Part model, mm, in its own coordinate system. A direction names the side the tool comes from. Coordinates: 2 decimals unless noted, no trailing zeros. Order: outer loops, then holes, each group sorted by start corner. A loop starts at its lowest first (then second) coordinate and runs counter-clockwise, first axis right, second up.
from build123d import *

# Parameters (mm, degrees)
BOSS_EXTRUDE1_DEPTH               = 2
BOSS_EXTRUDE2_DEPTH               = 4
BOSS_EXTRUDE3_DEPTH               = 1
BOSS_EXTRUDE4_DEPTH               = 3
SKETCH7_W                         = 13
SKETCH7_H                         = 25
CUT_EXTRUDE2_DEPTH                = 0.75
F_3_0_3_DIAMETER_HOLE1_D          = 3
SKETCH12_W                        = 0.5
SKETCH12_H                        = 1.222432211
F_1_0_1_DIAMETER_HOLE1_AT_2_COUNT = 2
F_1_0_1_DIAMETER_HOLE1_AT_2_PITCH = 2
F_1_0_1_DIAMETER_HOLE2_D          = 1
F_1_0_1_DIAMETER_HOLE2_DEPTH      = 3
SKETCH18_W                        = 25
SKETCH18_H                        = 13
CUT_EXTRUDE4_DEPTH                = 10
SKETCH19_W                        = 25
SKETCH19_H                        = 13
CUT_EXTRUDE5_DEPTH                = 62.758096635
SKETCH20_W                        = 0.67
SKETCH20_H                        = 16.929710607
BOSS_EXTRUDE5_DEPTH               = 3
F_1_0_1_DIAMETER_HOLE3_D          = 1
F_1_0_1_DIAMETER_HOLE3_DEPTH      = 3


with BuildPart() as part:
    # Sketch1 → Boss-Extrude1 (new body)
    with BuildSketch(Plane(origin=(0, 0, 0), x_dir=(1, 0, 0), z_dir=(0, 1, 0))):
        Polygon((17.5, 42.5), (-39, 42.5), (-39, 17.5), (-44.5, 17.5), (-44.5, -17.5), (-39, -17.5), (-39, -42.5), (17.5, -42.5), (39, -42.5), (39, -17.5), (44.5, -17.5), (44.5, 17.5), (39, 17.5), (39, 42.5), align=None)
    extrude(amount=BOSS_EXTRUDE1_DEPTH)

    # Sketch2 → Boss-Extrude2 (add)
    with BuildSketch(Plane(origin=(0, 2, 0), x_dir=(1, 0, 0), z_dir=(0, 1, 0))):
        with BuildLine():
            Line((34.546315587, 23.429710607), (34.546315587, 0))
            Line((34.546315587, 0), (33.546315587, 0))
            Line((33.546315587, 0), (33.546315587, 23.429710607))
            ThreePointArc((33.546315587, 23.429710607), (33.151002872, 25.378262634), (32.027573585, 27.018699705))
            ThreePointArc((32.027573585, 27.018699705), (-1.976971125, 39.957497595), (-34.744767591, 24.14632855))
            Line((-34.744767591, 24.14632855), (-34.744767591, 25.651242078))
            ThreePointArc((-34.744767591, 25.651242078), (-1.451938229, 40.977567789), (32.723825185, 27.736497525))
            ThreePointArc((32.723825185, 27.736497525), (34.071940329, 25.76797304), (34.546315587, 23.429710607))
        make_face()
        with BuildLine():
            Line((33.55, -26.915004177), (33.55, -25.470581501))
            ThreePointArc((33.55, -25.470581501), (1.082760633, -39.987255076), (-32.031707317, -27.014689554))
            ThreePointArc((-32.031707317, -27.014689554), (-33.154809257, -25.374400109), (-33.55, -23.426136342))
            Line((-33.55, -23.426136342), (-33.55, 0))
            Line((-33.55, 0), (-34.55, 0))
            Line((-34.55, 0), (-34.55, -23.426136342))
            ThreePointArc((-34.55, -23.426136342), (-34.075771108, -25.764052863), (-32.72804878, -27.732400197))
            ThreePointArc((-32.72804878, -27.732400197), (0.579599012, -40.996426087), (33.55, -26.915004177))
        make_face()
    extrude(amount=BOSS_EXTRUDE2_DEPTH)

    # Sketch3 → Boss-Extrude3 (add)
    with BuildSketch(Plane(origin=(0, 2, 0), x_dir=(1, 0, 0), z_dir=(0, 1, 0))):
        with BuildLine():
            Line((-35.546315587, 42), (35.546315587, 42))
            Line((35.546315587, 42), (35.546315587, 0))
            Line((35.546315587, 0), (34.546315587, 0))
            Line((34.546315587, 0), (34.546315587, 23.446970837))
            ThreePointArc((34.546315587, 23.446970837), (34.071801154, 25.777287901), (32.723825185, 27.736497525))
            ThreePointArc((32.723825185, 27.736497525), (-1.450164751, 40.920186771), (-34.744767591, 25.651242078))
            Line((-34.744767591, 25.651242078), (-34.744767591, 24.14632855))
            Line((-34.744767591, 24.14632855), (-35.546315587, 24.14632855))
            Line((-35.546315587, 24.14632855), (-35.546315587, 25.914938844))
            Line((-35.546315587, 25.914938844), (-35.546315587, 42))
        make_face()
        with BuildLine():
            Line((-35.55, -42), (34.55, -42))
            Line((34.55, -42), (34.55, -25.470581501))
            Line((34.55, -25.470581501), (33.55, -25.470581501))
            Line((33.55, -25.470581501), (33.55, -26.915004177))
            ThreePointArc((33.55, -26.915004177), (0.579599012, -40.996426087), (-32.72804878, -27.732400197))
            ThreePointArc((-32.72804878, -27.732400197), (-34.075771108, -25.764052863), (-34.55, -23.426136342))
            Line((-34.55, -23.426136342), (-34.55, 0))
            Line((-34.55, 0), (-35.55, 0))
            Line((-35.55, 0), (-35.55, -42))
        make_face()
    extrude(amount=BOSS_EXTRUDE3_DEPTH)

    # Sketch4 → Boss-Extrude4 (add)
    with BuildSketch(Plane(origin=(0, 3, 0), x_dir=(1, 0, 0), z_dir=(0, 1, 0))):
        Polygon((5, 41.977567789), (-5.8, 41.977567789), (-5.8, 40.077567789), (-5, 40.077567789), (-5, 41.277567789), (5, 41.277567789), align=None)
    extrude(amount=BOSS_EXTRUDE4_DEPTH)

    # Sketch7 → Cut-Extrude2 (cut)
    with BuildSketch(Plane.XZ):
        with Locations((0, -25.5)):
            Rectangle(SKETCH7_W, SKETCH7_H)
        with Locations((0, 25.5)):
            Rectangle(SKETCH7_W, SKETCH7_H)
    extrude(amount=-CUT_EXTRUDE2_DEPTH, mode=Mode.SUBTRACT)

    # Ø3.0 (3) Diameter Hole1 (through all)
    with Locations(Plane(origin=(0, 2, 0), x_dir=(1, 0, 0), z_dir=(0, 1, 0))):
        with Locations((-23, 25), (-23, -25), (23, -25), (23, 25), (0, 0)):
            Hole(F_3_0_3_DIAMETER_HOLE1_D / 2)

    # Sketch12 → Ø1.0 (1) Diameter Hole1 (revolve, cut)
    with BuildSketch(Plane(origin=(-3.7, 4.5, -41.277567789), x_dir=(0, -1, 0), z_dir=(1, 0, 0))):
        with Locations((0.25, 0.611216106)):
            Rectangle(SKETCH12_W, SKETCH12_H)
    f_1_0_1_diameter_hole1 = revolve(axis=Axis((-3.7, 4.5, -34.927567789), (0, 0, -1)), mode=Mode.SUBTRACT)

    # Ø1.0 (1) Diameter Hole1 at 2: Ø1.0 (1) Diameter Hole1 ×2
    with Locations(*[(i * F_1_0_1_DIAMETER_HOLE1_AT_2_PITCH, 0, 0) for i in range(1, F_1_0_1_DIAMETER_HOLE1_AT_2_COUNT)]):
        add(f_1_0_1_diameter_hole1, mode=Mode.SUBTRACT)

    # Ø1.0 (1) Diameter Hole2
    with Locations(Plane.ZY.offset(-33.546315587)):
        with Locations((-19.169710607, 4.5), (-16.169710607, 4.5)):
            Hole(F_1_0_1_DIAMETER_HOLE2_D / 2, depth=F_1_0_1_DIAMETER_HOLE2_DEPTH)

    # Sketch18 → Cut-Extrude4 (cut)
    with BuildSketch(Plane.XZ.offset(-0.75)):
        with Locations((-25.5, 0)):
            Rectangle(SKETCH18_W, SKETCH18_H)
        with Locations((25.5, 0)):
            Rectangle(SKETCH18_W, SKETCH18_H)
    extrude(amount=-CUT_EXTRUDE4_DEPTH, mode=Mode.SUBTRACT)

    # Sketch19 → Cut-Extrude5 (cut, through all)
    with BuildSketch(Plane(origin=(0, 0.75, 0), x_dir=(1, 0, 0), z_dir=(0, 1, 0))):
        with Locations((-25.5, 0)):
            Rectangle(SKETCH19_W, SKETCH19_H)
        with Locations((25.5, 0)):
            Rectangle(SKETCH19_W, SKETCH19_H)
    extrude(amount=-CUT_EXTRUDE5_DEPTH, mode=Mode.SUBTRACT)

    # Sketch20 → Boss-Extrude5 (add)
    with BuildSketch(Plane(origin=(0, 3, 0), x_dir=(1, 0, 0), z_dir=(0, 1, 0))):
        with Locations((35.211315587, 14.964855304)):
            Rectangle(SKETCH20_W, SKETCH20_H)
    extrude(amount=BOSS_EXTRUDE5_DEPTH)

    # Ø1.0 (1) Diameter Hole3
    with Locations(Plane.ZY.offset(-34.876315587)):
        with Locations((-19.169710607, 4.5), (-16.169710607, 4.5)):
            Hole(F_1_0_1_DIAMETER_HOLE3_D / 2, depth=F_1_0_1_DIAMETER_HOLE3_DEPTH)


solid = part.part
Q1. Mould opens along Z. For faces 5 (the face through (44.5, 1, 0)), 6 (the face through (42, 1, 17.5)), 7 (the face through (-22.805, 0.986, -26.487)) say: pulls with the +Z half, pulls with the -Z half, needs draft (parallel to the pull), parting line crosses it, or undercut.
Results list:
face 5: needs draft
face 6: pulls with the +Z half
face 7: undercut
Q2. Cut at B-B on z = 8.5. Write the cut outline in (x, y), and give its area (3 significant figures).
Results list:
outline: (-44.5, 0) - (44.5, 0) - (44.5, 2) - (-33.55, 2) - (-33.55, 6) - (-34.55, 6) - (-34.55, 3) - (-35.55, 3) - (-35.55, 2) - (-44.5, 2) - close
area: 183 mm2
Q3. Cut at C-C on x = -23. Write the cut outline in (y, z), and give its area (3 significant figures).
Results list:
outline: (0, -42.5) - (2, -42.5) - (2, -42) - (3, -42) - (3, -34.99) - (6, -34.99) - (6, -33.84) - (2, -33.84) - (2, -26.5) - (0, -26.5) - close; (0, -23.5) - (2, -23.5) - (2, -6.5) - (0, -6.5) - close; (0, 6.5) - (2, 6.5) - (2, 23.5) - (0, 23.5) - close; (0, 26.5) - (2, 26.5) - (2, 33.84) - (6, 33.84) - (6, 34.99) - (3, 34.99) - (3, 42) - (2, 42) - (2, 42.5) - (0, 42.5) - close
area: 155 mm2
Q4. Wall check: line 1 along X through (y, z) = (4.5, -41.6); line 2 along Z through (x, y) = (-23, 0.95); line 3 along Y through (x, z) = (39, 7.5). Give the ranges that are in metal, low to high.
Results list:
line 1: x = -5.8 to -4.2, -3.2 to -2.2, -1.2 to 5
line 2: z = -42.5 to -26.5, -23.5 to -6.5, 6.5 to 23.5, 26.5 to 42.5
line 3: y = 0 to 2
Q5. Which spindle directions (+Z, -Z, +X, -X, +Y, -Y) get a long thin tool onto all of the face, cutting with end or side? Do faces 1 (the face through (34.546, 4, -15)), 2 (the face through (33.546, 4, -15)), 3 (the face through (-3.3, 3, 41.3)), 4 (the face through (-39, 1, -30)). Say none if no direction does.
Results list:
face 1: +Z, -Z, +Y
face 2: -X, +Y
face 3: +Z, +Y
face 4: -Z, -X, +Y, -Y
Q6. Cut at D-D on z = 35. Write the cut outline in (x, y), and give its area (3 significant figures).
Results list:
outline: (-39, 0) - (-6.5, 0) - (-6.5, 0.75) - (6.5, 0.75) - (6.5, 0) - (39, 0) - (39, 2) - (34.55, 2) - (34.55, 3) - (22.98, 3) - (22.98, 6) - (20.86, 6) - (20.86, 2) - (-20.86, 2) - (-20.86, 6) - (-22.98, 6) - (-22.98, 3) - (-35.55, 3) - (-35.55, 2) - (-39, 2) - close
area: 187 mm2
Q7. Pin check, flat tips, straight feed: pin 1 Ø0.8 at (x, y) = (34, 2.5) entering from -Z; pin 2 Ø1.5 at (y, z) = (5, -18) entering from +X; pin 3 Ø1.5 at (x, z) = (16.5, 32.5) entering from +Y; pin 4 Ø3 at (x, z) = (-11, -30.5) entering from -Y. Stop position of each tip, or through.
Results list:
pin 1: stops at z = -42
pin 2: stops at x = 35.55
pin 3: stops at y = 2
pin 4: stops at y = 0
